Geometry check sheet. Reference: drawing and pictorial views, mm from the part's lowest x, y, z. A direction names the side the tool comes from. Coordinates: 2 decimals unless noted, no trailing zeros. Loops run counter-clockwise (first coordinate to the right, second up) from the corner with the lowest first, then second, coordinate; pieces in that order, holes last. Notation, with made-up numbers: (30, 46.5) -> (40, 46.5) arc R22 ccw to (40, 83.5) -> close; hole circle Ø7 at (-26.5, 10). An arc over 180 degrees is marked (long way). Use one line per item in the form item = value.
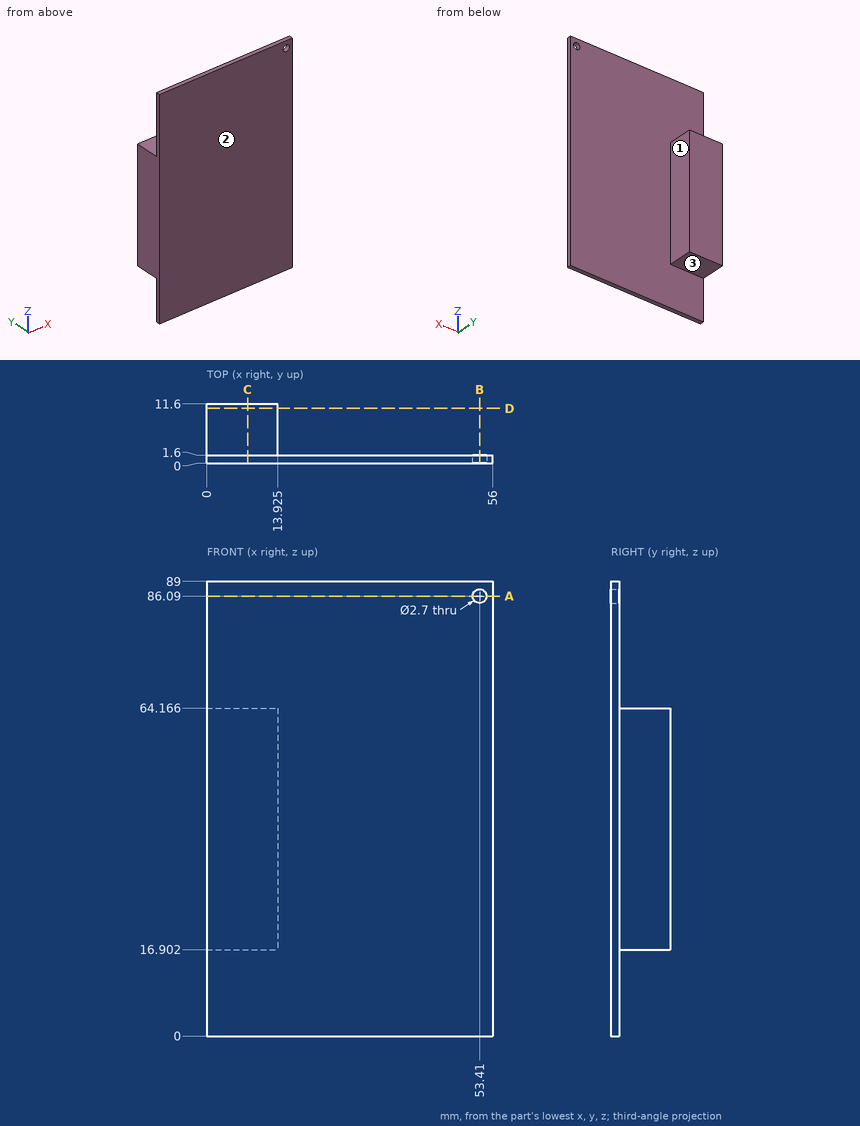
(1) Section check B-B, the plane x = 53.41. Record the boundary of the cut face in (y, z).
Established:
outline = (0, 0) -> (1.6, 0) -> (1.6, 84.74) -> (0, 84.74) -> close; (0, 87.44) -> (1.6, 87.44) -> (1.6, 89) -> (0, 89) -> close
(2) Tool access check on the marked faces 1, 2 and 3. Record the directions out of +Z, -Z, +X, -X, +Y, -Y that give a thin tool (end or side, any length) a straight path to the whole face; none if there is none.
Established:
face_1 = +Z, -Z, +X, +Y
face_2 = +Z, -Z, +X, -X, -Y
face_3 = -Z, +X, -X, +Y
(3) Section check D-D, the plane y = 10.75. Record the boundary of the cut face in (x, z) (1 decimal).
Established:
outline = (0, 16.9) -> (13.9, 16.9) -> (13.9, 64.2) -> (0, 64.2) -> close
(4) Section check C-C, the plane x = 8. Record the boundary of the cut face in (y, z).
Established:
outline = (0, 0) -> (1.6, 0) -> (1.6, 16.9) -> (11.6, 16.9) -> (11.6, 64.17) -> (1.6, 64.17) -> (1.6, 89) -> (0, 89) -> close
(5) Scan lines: line 1 along X through (y, z) = (0.75, 86.09); line 2 along Z through (x, y) = (53.41, 0.75); line 3 along Z through (x, y) = (7, 7). Record each from-to range of solid material in increasing order.
Established:
line_1 = 0 to 52.06, 54.76 to 56
line_2 = 0 to 84.74, 87.44 to 89
line_3 = 16.9 to 64.17
(6) Go/stop test with flat-tipped pins: P1, Ø2, axis at x = 53.41, z = 86.09, coming from the +Y side; P2, Ø1.5, axis at x = 24, z = 67.5, coming from the +Y side; P3, Ø3, axis at y = 5, z = 41, coming from the +X side (3 decimals). Record where each tip stops, or that it passes through.
Established:
P1 = through
P2 = 1.6
P3 = 13.925
(7) Section check A-A, the plane z = 86.09. Record the boundary of the cut face in (x, y).
Established:
outline = (0, 0) -> (52.06, 0) -> (52.06, 1.6) -> (0, 1.6) -> close; (54.76, 0) -> (56, 0) -> (56, 1.6) -> (54.76, 1.6) -> close
